Geometry check sheet. Reference: drawing and pictorial views, mm from the part's lowest x, y, z. A direction names the side the tool comes from. Give positions to 0.01 mm unless a question says otherwise; leave off trailing zeros. Loops run counter-clockwise (first coordinate to the right, second up) from the corner with the lowest first, then second, coordinate; pieces in that order, holes last. Notation, with made-up numbers: (-5.75, -19) -> (27.25, -19) arc R10 cw to (27.25, -8) -> close; hole circle Ø11 at (71, 36.25). An arc over 180 degrees is marked (long way). One line per item, written item: value. Start each with the question number.
(1) Sectioned sample at C-C, the plane x = 8.5. State how many separate pieces and enclosed holes the cut face has, then the cut area to 4 significant figures.
(2) Sectioned sample at B-B, the plane z = 22.5. Record the cut outline in (x, y).
(3) Scan lines: line 1 along Y through (x, z) = (8.5, 1.25); line 2 along Z through (x, y) = (8.5, 0.5); line 3 along Z through (x, y) = (4, 13). Record each from-to range of solid material in increasing order. Write a range as from..to.
(4) Sectioned sample at D-D, the plane x = 10.75. Record the cut outline in (y, z), then the cut area to 4 significant figures.
(5) Tool access check on the marked faces 1 and 2. Record the directions out of +Z, -Z, +X, -X, +Y, -Y that give a thin tool (end or side, any length) a straight path to the whole face; none if there is none.
(6) Gauge pin test, flat ends, axial feed: pin 1 Ø3 at (x, z) = (3.5, 20.5) entering from +Y; pin 2 Ø1.8 at (x, z) = (8.5, 10.5) entering from -Y; pin 3 Ø3 at (x, y) = (8.5, 10.5) entering from -Z; pin 4 Ø4 at (x, y) = (8.5, 17) entering from +Z. Record the tip position at first contact, or that the pin passes through.
(7) Sectioned sample at A-A, the plane y = 17. Record the cut outline in (x, z), then the cut area to 3 significant figures.
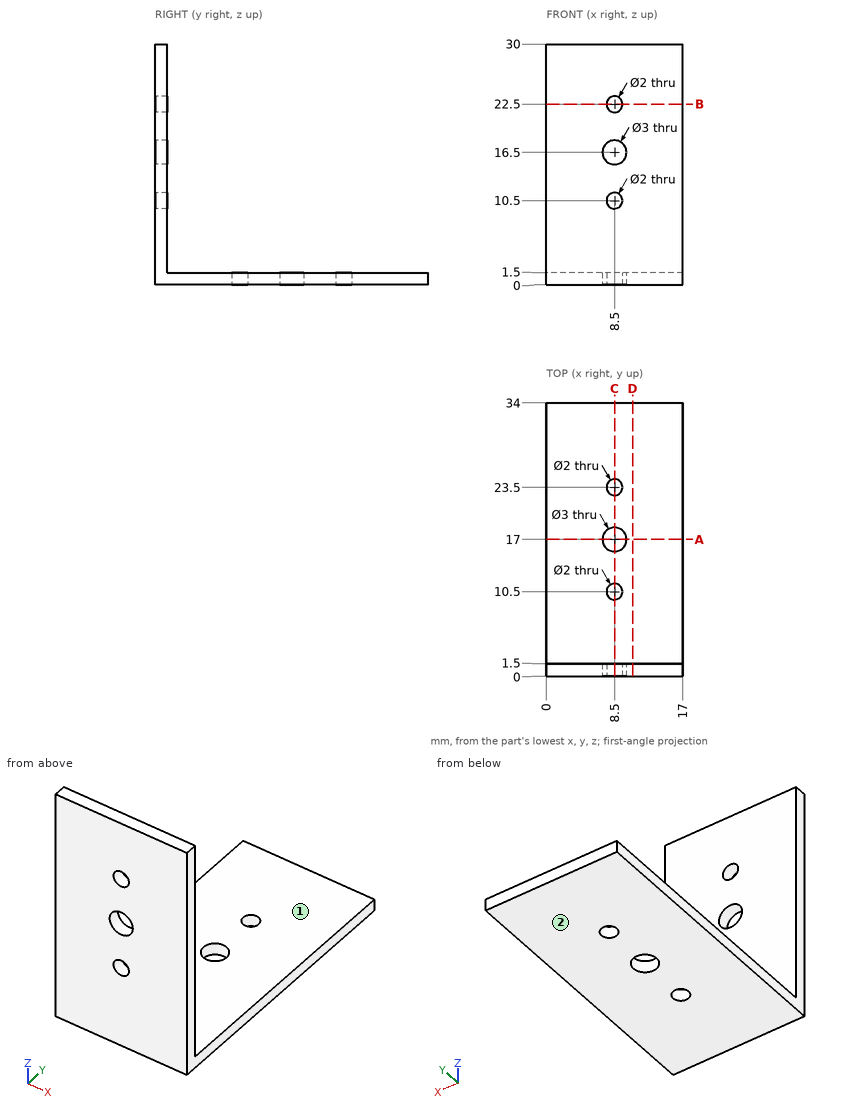
Calculated:
1. separate pieces: 7
1. enclosed holes: 0
1. area: 72.75 mm2
2. outline: (0, 0) -> (7.5, 0) -> (7.5, 1.5) -> (0, 1.5) -> close; (9.5, 0) -> (17, 0) -> (17, 1.5) -> (9.5, 1.5) -> close
3. line 1: y = 0..9.5, 11.5..15.5, 18.5..22.5, 24.5..34
3. line 2: z = 0..9.5, 11.5..15, 18..21.5, 23.5..30
3. line 3: z = 0..1.5
4. outline: (0, 0) -> (34, 0) -> (34, 1.5) -> (1.5, 1.5) -> (1.5, 30) -> (0, 30) -> close
4. area: 93.75 mm2
5. face 1: +Z, +X, -X, +Y
5. face 2: -Z, +X, -X, +Y, -Y
6. pin 1: stops at y = 1.5
6. pin 2: passes through
6. pin 3: stops at z = 0
6. pin 4: stops at z = 1.5
7. outline: (0, 0) -> (7, 0) -> (7, 1.5) -> (0, 1.5) -> close; (10, 0) -> (17, 0) -> (17, 1.5) -> (10, 1.5) -> close
7. area: 21.0 mm2
